```python
from build123d import *

# Parameters (mm, degrees)
BOX002_W          = 4.5
BOX002_H          = 29
BOX002_DEPTH      = 10
CYLINDER003_R     = 14.5
CYLINDER003_DEPTH = 5.5
CYLINDER002_R     = 3.9
CYLINDER002_DEPTH = 10
CYLINDER_R        = 13.75
CYLINDER_DEPTH    = 49.6
BOX_W             = 36
BOX_H             = 36
BOX_DEPTH         = 4
BOX001_W          = 10
BOX001_H          = 10
BOX001_DEPTH      = 10
CYLINDER001_R     = 16.32
CYLINDER001_DEPTH = 52


with BuildPart() as cube002:
    # Box002 → Box002 (new body)
    with BuildSketch(Plane(origin=(-2.2, -14.46, 0), x_dir=(1, 0, 0), z_dir=(0, 0, 1))):
        with Locations((2.25, 14.5)):
            Rectangle(BOX002_W, BOX002_H)
    extrude(amount=BOX002_DEPTH)


with BuildPart() as cylinder003:
    # Cylinder003 → Cylinder003 (new body)
    with BuildSketch(Plane.XY.offset(2.1)):
        Circle(CYLINDER003_R)
    extrude(amount=CYLINDER003_DEPTH)


with BuildPart() as cylinder002:
    # Cylinder002 → Cylinder002 (new body)
    with BuildSketch(Plane(origin=(-20, 0, 43), x_dir=(0, 0, -1), z_dir=(1, 0, 0))):
        Circle(CYLINDER002_R)
    extrude(amount=CYLINDER002_DEPTH)


with BuildPart() as cylinder:
    # Cylinder → Cylinder (new body)
    with BuildSketch(Plane.XY):
        Circle(CYLINDER_R)
    extrude(amount=CYLINDER_DEPTH)


with BuildPart() as cube:
    # Box → Box (new body)
    with BuildSketch(Plane(origin=(-18, -18, 48), x_dir=(1, 0, 0), z_dir=(0, 0, 1))):
        with Locations((18, 18)):
            Rectangle(BOX_W, BOX_H)
    extrude(amount=BOX_DEPTH)


with BuildPart() as cube001:
    # Box001 → Box001 (new body)
    with BuildSketch(Plane(origin=(-18, -5, 38), x_dir=(1, 0, 0), z_dir=(0, 0, 1))):
        with Locations((5, 5)):
            Rectangle(BOX001_W, BOX001_H)
    extrude(amount=BOX001_DEPTH)


with BuildPart() as cut003:
    # Cylinder001 → Cylinder001 (new body)
    with BuildSketch(Plane.XY):
        Circle(CYLINDER001_R)
    extrude(amount=CYLINDER001_DEPTH)

    # Fusion: union Cube, Cube001
    add(cube.part)
    add(cube001.part)

    # Cut: cut Cylinder
    add(cylinder.part, mode=Mode.SUBTRACT)

    # Cut001: cut Cylinder002
    add(cylinder002.part, mode=Mode.SUBTRACT)

    # Cut002: cut Cylinder003
    add(cylinder003.part, mode=Mode.SUBTRACT)

    # Cut003: cut Cube002
    add(cube002.part, mode=Mode.SUBTRACT)


solid = cut003.part
```
Verification items for the finished model (mm, model axes). A direction names the side the tool comes from. Give positions to 0.01 mm unless a question says otherwise; leave off trailing zeros. Order: outer loops, then holes, each group sorted by start corner. A loop starts at its lowest first (then second) coordinate and runs counter-clockwise, first axis right, second up. Notation, with made-up numbers: (82, -8.75) - (126, -8.75) arc R22 cw to (126, 26.25) - close; hole circle Ø6 at (77.5, 68). An arc over 180 degrees is marked (long way). Answer as CSV lines item,"result". Start each with the question number.
Item 1: Section check C-C, the plane z = 8.5. Record the boundary of the cut face in (x, y).
Item 2: Section check D-D, the plane z = 43. Record the boundary of the cut face in (x, y), plus the area to 3 significant figures.
Item 3: Mould release check, pull along X, two halves, no side actions. Record for faces 1 (the face through (18, 0, 50)), 2 (the face through (0, 0, 49.6)), 3 (the face through (0, 0, 52)): released by +X, released by -X, zero draft, split by the parting line, or undercut.
Item 4: Material ranges on L1, parallel to Z at x = -14.35, y = 0; L2, parallel to Y at x = -16.85, z = 43; L3, parallel to Y at x = 0, z = 39.5, recorded low to high.
Item 5: Section check A-A, the plane y = 0. Record the boundary of the cut face in (x, z).
Item 6: Gauge pin test, flat ends, axial feed: pin 1 (4 mm diameter, centred on y = 0.5, z = 29, fed in from -X); pin 2 (2 mm diameter, centred on x = 5, z = 9.5, fed in from +Y); pin 3 (8 mm diameter, centred on x = -6.5, y = 5.5, fed in from -Z). Record the tip position at first contact, or that the pin passes through.
Item 7: Access from +Z, -Z, +X, -X, +Y, -Y to the whole of each face (thin tool, end or side, straight path). Record for faces 4 (the face through (2, -14.46, 5)), 5 (the face through (-15.6, -1.5, 39.4)), 6 (the face through (-17, 5, 43)), 7 (the face through (-14, 0, 2.1)), 8 (the face through (-17, -5, 43)).
Filled in:
1,outline,"circle Ø32.64 at (0, 0); hole (-2.2, -14.46) - (2.3, -14.46) - (2.3, -13.56) arc R13.75 ccw to (2.3, 13.56) - (2.3, 14.54) - (-2.2, 14.54) - (-2.2, 13.57) arc R13.75 ccw to (-2.2, -13.57) - close"
2,outline,"(-18, -5) - (-15.54, -5) arc R16.32 ccw (long way) to (-15.54, 5) - (-18, 5) - (-18, 3.9) - (-13.19, 3.9) arc R13.75 cw (long way) to (-13.19, -3.9) - (-18, -3.9) - close"
2,area,"228 mm^2"
3,face 1,"released by +X"
3,face 2,"undercut"
3,face 3,"zero draft"
4,L1,"0 to 2.1, 7.6 to 39.1, 46.9 to 52"
4,L2,"-5 to -3.9, 3.9 to 5"
4,L3,"-16.32 to -13.75, 13.75 to 16.32"
5,outline,"(-18, 38) - (-16.32, 38) - (-16.32, 0) - (-13.75, 0) - (-13.75, 2.1) - (-14.5, 2.1) - (-14.5, 7.6) - (-13.75, 7.6) - (-13.75, 39.1) - (-18, 39.1) - close; (-18, 46.9) - (-13.75, 46.9) - (-13.75, 49.6) - (13.75, 49.6) - (13.75, 7.6) - (14.5, 7.6) - (14.5, 2.1) - (13.75, 2.1) - (13.75, 0) - (16.32, 0) - (16.32, 48) - (18, 48) - (18, 52) - (-18, 52) - close"
6,pin 1,"x = -16.32"
6,pin 2,"y = 15.82"
6,pin 3,"z = 49.6"
7,face 4,"-Z"
7,face 5,"-X"
7,face 6,"-Z, -X, +Y"
7,face 7,"none"
7,face 8,"-Z, -X, -Y"
